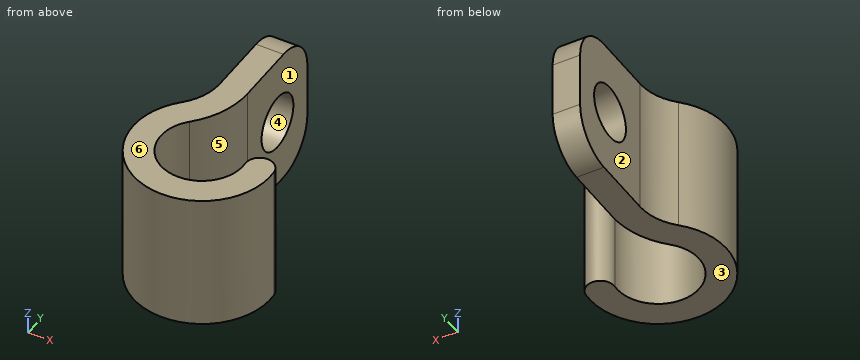
from build123d import *

# Parameters (mm, degrees)
F1_DEPTH = 10
F2_R     = 3
F4_D     = 4


with BuildPart() as f1:
    # F0 (on Top) → F1 (new body)
    with BuildSketch(Plane.XY):
        with BuildLine():
            ThreePointArc((3.352545125, -13.6172124282), (-0.6620993993, -16.6977575188), (-1.7573593129, -11.7573593129))
            ThreePointArc((-1.7573593129, -11.7573593129), (-0.4567228049, -9.81081922), (0, -7.5147186258))
            Line((0, -7.5147186258), (0, 0))
            Line((0, 0), (-2, 0))
            Line((-2, 0), (-2, -7.5147186258))
            ThreePointArc((-2, -7.5147186258), (-2.30448187, -9.0454523552), (-3.1715728753, -10.3431457505))
            ThreePointArc((-3.1715728753, -10.3431457505), (-1.3461396859, -18.5771427604), (5.3449345211, -13.4429009427))
            ThreePointArc((5.3449345211, -13.4429009427), (4.2615840803, -12.5338619874), (3.352545125, -13.6172124282))
        make_face()
    extrude(amount=F1_DEPTH)

    # F2
    f2_edges = [f1.edges().sort_by_distance(p)[0] for p in [
        (-1, 0, 10),
        (-1, 0, 0),
    ]]
    fillet(f2_edges, radius=F2_R)

    # F4 (through all)
    with Locations(Plane.YZ):
        with Locations((-3.7573593129, 5)):
            Hole(F4_D / 2)


solid = f1.part
Verification items for the finished model (mm, model axes). Face numbers are marked on the shaded views. A direction names the side the tool comes from. Coordinates: 2 decimals unless noted, no trailing zeros. Loops run counter-clockwise (first coordinate to the right, second up) from the corner with the lowest first, then second, coordinate; pieces in that order, holes last. Notation, with made-up numbers: (9, -12.75) -> (26, -12.75) arc R25 cw to (26, 5.25) -> close; hole circle Ø4 at (-23.5, 66.25). An arc over 180 degrees is marked (long way). Answer as a JSON object with one key per item and string values. Group by question number.
Item 1: Sectioned sample at B-B on y = -2. Record the boundary of the cut face in (x, z).
Item 2: Mould release check, pull along Z, two halves, no side actions. Record for the marked faces 4, 5 and 6: +Z half, -Z half, draft (parallel to the pull), parting line (faces both ways), or undercut.
Item 3: Tool access check on the marked faces 1, 2 and 3. Record the directions out of +Z, -Z, +X, -X, +Y, -Y that give a thin tool (end or side, any length) a straight path to the whole face; none if there is none.
Item 4: Sectioned sample at C-C on x = -1. Record the boundary of the cut face in (y, z).
Item 5: Sectioned sample at A-A on z = 6.25. Record the boundary of the cut face in (x, y).
Item 6: Scan lines: probe 1 along Y at (x, z) = (-1, 5.75); probe 2 along X at (y, z) = (-2, 7.25); probe 3 along Y at (x, z) = (-1, 7.75). Record each from-to range of solid material in increasing order.
Item 7: Depth check by flat-ended pin: pin 1 (1 mm diameter, centred on x = 3.5, z = 8, fed in from +Y); pin 2 (2.5 mm diameter, centred on y = -2.5, z = 5, fed in from -X); pin 3 (6 mm diameter, centred on y = -7, z = 6.5, fed in from -X). Enter the tip coordinate at first touch or a pass-through.
Item 8: Sectioned sample at D-D on z = 8.75. Record the boundary of the cut face in (x, y).
Evaluation:
{
 "1": {"outline": "(-2, 0.17) -> (0, 0.17) -> (0, 4.05) -> (-2, 4.05) -> close; (-2, 5.95) -> (0, 5.95) -> (0, 9.83) -> (-2, 9.83) -> close"},
 "2": {"face 4": "undercut", "face 5": "draft", "face 6": "+Z half"},
 "3": {"face 1": "+Z, -Z, +X, +Y", "face 2": "+Z, -Z, -X, +Y", "face 3": "-Z, +X, -X, +Y, -Y"},
 "4": {"outline": "(-18.69, 0) -> (-16.55, 0) -> (-16.55, 10) -> (-18.69, 10) -> close; (-10.83, 0) -> (-3, 0) arc R3 ccw to (0, 3) -> (0, 7) arc R3 ccw to (-3, 10) -> (-10.83, 10) -> close; hole circle Ø4 at (-3.76, 5)"},
 "5": {"outline": "(-3.17, -10.34) arc R5 ccw (long way) to (5.34, -13.44) arc R1 ccw to (3.35, -13.62) arc R3 cw (long way) to (-1.76, -11.76) arc R6 ccw to (0, -7.51) -> (0, -5.32) -> (-2, -5.32) -> (-2, -7.51) arc R4 cw to start; (-2, -2.2) -> (0, -2.2) -> (0, 0) -> (-2, 0) -> close"},
 "6": {"probe 1": "y = -18.69 to -16.55, -10.83 to -5.61, -1.9 to 0", "probe 2": "x = -2 to 0", "probe 3": "y = -18.69 to -16.55, -10.83 to -0.1"},
 "7": {"pin 1": "stops at y = -12.59", "pin 2": "stops at x = -2", "pin 3": "stops at x = -2.87"},
 "8": {"outline": "(-3.17, -10.34) arc R5 ccw (long way) to (5.34, -13.44) arc R1 ccw to (3.35, -13.62) arc R3 cw (long way) to (-1.76, -11.76) arc R6 ccw to (0, -7.51) -> (0, -0.56) -> (-2, -0.56) -> (-2, -7.51) arc R4 cw to start"}
}
